```python
from build123d import *

# Parameters (mm, degrees)
SKETCH1_R           = 1.5
SKETCH1_W           = 11.1125
SKETCH1_H           = 136.525
BOSS_EXTRUDE1_DEPTH = 1.5875


with BuildPart() as part:
    # Sketch1 → Boss-Extrude1 (new body)
    # profile 1 of 4: a face of its own
    with BuildSketch(Plane.XY):
        with BuildLine():
            ThreePointArc((-11.1125, 68.2625), (0, 79.375), (11.1125, 68.2625))
            Line((11.1125, 68.2625), (-11.1125, 68.2625))
        make_face()
        with Locations((0, 69.85)):
            Circle(SKETCH1_R, mode=Mode.SUBTRACT)
    # profile 2 of 4: a face of its own
    with BuildSketch(Plane.XY):
        with Locations((5.55625, 0)):
            Rectangle(SKETCH1_W, SKETCH1_H)
    # profile 3 of 4: a face of its own
    with BuildSketch(Plane.XY):
        with Locations((-5.55625, 0)):
            Rectangle(SKETCH1_W, SKETCH1_H)
    # profile 4 of 4: a face of its own
    with BuildSketch(Plane.XY):
        with BuildLine():
            Line((-11.1125, -68.2625), (11.1125, -68.2625))
            ThreePointArc((11.1125, -68.2625), (0, -79.375), (-11.1125, -68.2625))
        make_face()
        with Locations((0, -69.85)):
            Circle(SKETCH1_R, mode=Mode.SUBTRACT)
    extrude(amount=BOSS_EXTRUDE1_DEPTH)


solid = part.part
```
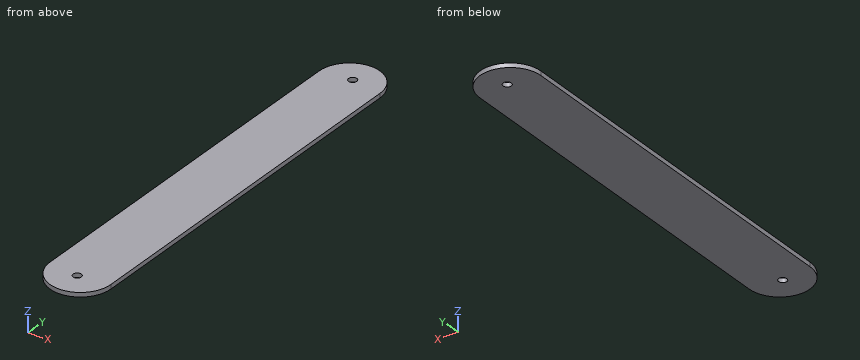
Input: part model. Units: mm. Frame: model coordinates. Round coordinates to 2 decimals unless told otherwise and drop trailing zeros. Loops run counter-clockwise (first coordinate to the right, second up) from the corner with the lowest first, then second, coordinate; pieces in that order, holes last.
1) Material intervals for line 1 (Y direction, x = 0, z = 0.65) (3 decimals); line 2 (Y direction, x = -1.25, z = 1.45); line 3 (X direction, y = -68.5, z = 1.15), sorted ascending.
Ans:
line 1: y = -79.375 to -71.35, -68.35 to 68.35, 71.35 to 79.375
line 2: y = -79.3 to -70.68, -69.02 to 69.02, 70.68 to 79.3
line 3: x = -11.11 to -0.65, 0.65 to 11.11
2) Section query C-C on y = -69.85. Return the cut outline in (x, z).
Ans:
outline: (-11, 0) - (-1.5, 0) - (-1.5, 1.59) - (-11, 1.59) - close; (1.5, 0) - (11, 0) - (11, 1.59) - (1.5, 1.59) - close
3) Section query D-D on x = -8. Return the cut outline in (y, z).
Ans:
outline: (-75.98, 0) - (75.98, 0) - (75.98, 1.59) - (-75.98, 1.59) - close
4) Section query A-A on z = 0.85. Count the separate pieces of the cut face and the enclosed holes in it, plus the area to 3 significant figures.
Ans:
separate pieces: 1
enclosed holes: 2
area: 3,410 mm2
